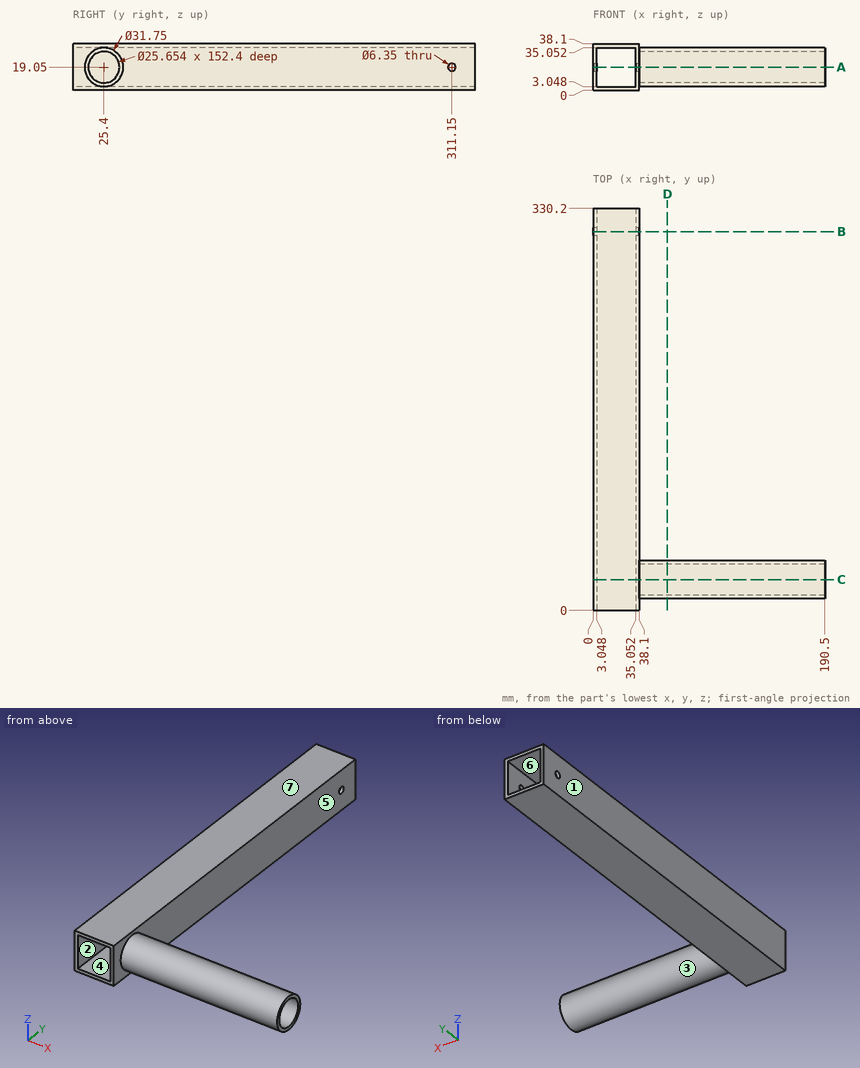
Can you work these out from the drawing? Everything is in mm from the part's minimum corner. A direction names the side the tool comes from. Round coordinates to 2 decimals unless told otherwise and drop trailing zeros. Order: outer loops, then holes, each group sorted by start corner. A loop starts at its lowest first (then second) coordinate and runs counter-clockwise, first axis right, second up. Notation, with made-up numbers: (26.25, -18) -> (42.25, -18) arc R15 cw to (42.25, 8) -> close; hole circle Ø10 at (8, 26). An arc over 180 degrees is marked (long way). Use CSV: the item, a comma, the result in double quotes.
1. I'm going to push flat-ended pins straight in: P1, Ø5.5, axis at y = 311.15, z = 19.05, coming from the +X side; P2, Ø2, axis at y = 58.5, z = 32.5, coming from the +X side; P3, Ø10, axis at x = 134.5, z = 12, coming from the +Y side. Where does each tip first touch, or does it pass through?
Recorded:
P1,"passes through"
P2,"stops at x = 38.1"
P3,"stops at y = 41.14"
2. I need wall thicknesses on line 1 along X through (y, z) = (61, 28); line 2 along Z through (x, y) = (94, 25). Which ranges of each line are inside material? Lowest first, please.
Recorded:
line 1,"x = 0 to 3.05, 35.05 to 38.1"
line 2,"z = 3.18 to 6.23, 31.87 to 34.92"
3. Thinking about a two-plate mould opening in X: for the marked faces 4, 5, 6 and 7, which applies, pulls with the +X half, pulls with the -X half, needs draft (parallel to the pull), parting line crosses it, or undercut?
Recorded:
face 4,"undercut"
face 5,"pulls with the +X half"
face 6,"undercut"
face 7,"needs draft"
4. I want a section at A-A on z = 19.05. List the corners of the cut face in (x, y) for me (3 decimals), and give its area (3 significant figures).
Recorded:
outline,"(0, 0) -> (3.048, 0) -> (3.048, 307.975) -> (0, 307.975) -> close; (0, 314.325) -> (3.048, 314.325) -> (3.048, 330.2) -> (0, 330.2) -> close; (35.052, 0) -> (38.1, 0) -> (38.1, 9.525) -> (190.5, 9.525) -> (190.5, 12.573) -> (38.1, 12.573) -> (38.1, 38.227) -> (190.5, 38.227) -> (190.5, 41.275) -> (38.1, 41.275) -> (38.1, 307.975) -> (35.052, 307.975) -> close; (35.052, 314.325) -> (38.1, 314.325) -> (38.1, 330.2) -> (35.052, 330.2) -> close"
area,"2,900 mm2"
5. I want a section at C-C on y = 25.4. List the corners of the cut face in (x, z) for me (3 decimals).
Recorded:
outline,"(0, 0) -> (38.1, 0) -> (38.1, 3.175) -> (190.5, 3.175) -> (190.5, 6.223) -> (38.1, 6.223) -> (38.1, 31.877) -> (190.5, 31.877) -> (190.5, 34.925) -> (38.1, 34.925) -> (38.1, 38.1) -> (0, 38.1) -> close; hole (3.048, 3.048) -> (35.052, 3.048) -> (35.052, 35.052) -> (3.048, 35.052) -> close"
6. Which directions (+Z, -Z, +X, -X, +Y, -Y) give clear straight access to the entire face, cutting with the end or side of a thin tool? Please do the marked faces 1, 2 and 3.
Recorded:
face 1,"+Z, -Z, -X, +Y, -Y"
face 2,"+Y, -Y"
face 3,"+X"
7. I want a section at B-B on y = 311.15. List the corners of the cut face in (x, z) for me (3 decimals), and give its area (3 significant figures).
Recorded:
outline,"(0, 0) -> (38.1, 0) -> (38.1, 15.875) -> (35.052, 15.875) -> (35.052, 3.048) -> (3.048, 3.048) -> (3.048, 15.875) -> (0, 15.875) -> close; (0, 22.225) -> (3.048, 22.225) -> (3.048, 35.052) -> (35.052, 35.052) -> (35.052, 22.225) -> (38.1, 22.225) -> (38.1, 38.1) -> (0, 38.1) -> close"
area,"389 mm2"
8. I want a section at D-D on x = 61. List the corners of the cut face in (y, z) for me (3 decimals).
Recorded:
outline,"circle Ø31.75 at (25.4, 19.05); hole circle Ø25.654 at (25.4, 19.05)"
